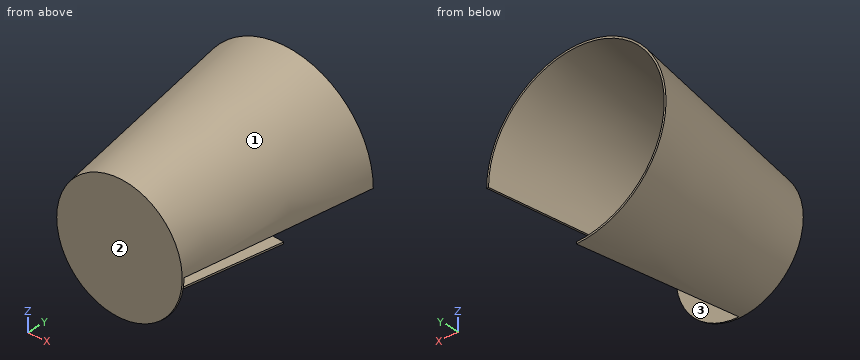
Autodesk Inventor part; units mm, degrees
ref_plane "Work Plane1" through (0, 260, 0) normal (0, 1, 0) x (-1, 0, 0)
ref_plane "YZ Plane" through (0, 0, 0) normal (1, 0, 0) x (0, 1, 0)
ref_plane "XY Plane" through (0, 0, 0) normal (0, 0, 1) x (1, 0, 0)
sketch "Sketch1" plane through (0, 0, 0) normal (0, 1, 0) x (-1, 0, 0)
  circle A0 centre (0, 0) radius 87.5
  dimension "d0" = 175
ref_plane "Work Plane1" through (0, 260, 0) normal (0, 1, 0) x (-1, 0, 0)
sketch "Sketch2" plane through (0, 260, 0) normal (0, 1, 0) x (-1, 0, 0)
  circle A0 centre (0, 0) radius 125
  dimension "d2" = 250
loft "Loft1" add profiles "Sketch1", "Sketch2"
shell "Shell1" thickness 2.5 removed faces 1 at (0.6944, 260, 22.8612)
sketch "Sketch3" plane through (0, 260, 0) normal (0, 1, 0) x (1, 0, 0)
  line L0 (0, 0) -> (156, 0)
  line L1 (0, 0) -> (0, 209)
  line L2 (0, 209) -> (156, 209)
  line L3 (156, 209) -> (156, 0)
extrude "Extrusion1" cut sketch "Sketch3" against normal up to surface (257.5 mm away)
properties part number "Topf" material "Concrete"
Check sheet for the modelled part. Datum: model origin and axes. Units: mm. Face numbers are marked on the shaded views. Coordinates: 2 decimals unless noted, no trailing zeros. Order: outer loops, then holes, each group sorted by start corner. A loop starts at its lowest first (then second) coordinate and runs counter-clockwise, first axis right, second up. Notation, with made-up numbers: M 84.25,57.5 L 136.25,57.5 A31 ccw 136.25,87.5 Z; hole C 70.25,64.5 d1. An arc over 180 degrees is marked long. Write each question's results on one line, items separated by ' | '. Start each with the question number.
1. Go/stop test with flat-tipped pins: P1, Ø10, axis at x = -91, y = 182, coming from the +Z side; P2, Ø4, axis at x = -35, z = -25, coming from the +Y side; P3, Ø5, axis at x = -72, z = 3.5, coming from the -Y side; P4, Ø1.5, axis at x = -60, y = 102, coming from the +Z side. Record where each tip stops, or that it passes through.
2. Cross-section at A-A on y = 210. Record the cut outline in (x, z), and give its area (3 significant figures).
3. Cross-section at B-B on y = 26. Record the cut outline in (x, z), and give its area (3 significant figures).
4. Material ranges on probe 1 along Z at (x, y) = (-78.5, 184); probe 2 along X at (y, z) = (194.5, 75.5); probe 3 along Y at (x, z) = (-11, 71), recorded low to high.
5. Mould release check, pull along Z, two halves, no side actions. Record for the marked faces 1, 2 and 3: +Z half, -Z half, draft (parallel to the pull), parting line (faces both ways), or undercut.
Checks:
1) P1: stops at z = 74.56 | P2: stops at y = 2.5 | P3: stops at y = 0 | P4: stops at z = 83.3
2) outline: M 0,-117.79 L 0,-115.26 A115.26 cw long 115.26,0 L 117.79,0 A117.79 ccw long Z | area: 1,390 mm²
3) outline: M 0,-91.25 L 0,-88.72 A88.72 cw long 88.72,0 L 91.25,0 A91.25 ccw long Z | area: 1,070 mm²
4) probe 1: z = -82.72 to -79.2, 79.2 to 82.72 | probe 2: x = -87.48 to -84.11, 84.11 to 87.48 | probe 3: y = 0 to 2.5
5) face 1: parting line | face 2: draft | face 3: undercut
